Design review of the part built by this model. Coordinates are the model's own, in mm. A direction names the side the tool comes from. Round coordinates to 2 decimals unless told otherwise and drop trailing zeros. Loops run counter-clockwise (first coordinate to the right, second up) from the corner with the lowest first, then second, coordinate; pieces in that order, holes last. Notation, with made-up numbers: (-3.5, 12.5) - (7.5, 12.5) arc R18 ccw to (7.5, 30.5) - close; hole circle Ø7 at (11, -31.75). An arc over 180 degrees is marked (long way). Return JSON: item names as keys, results as strings. Group by question number.
from build123d import *

# Parameters (mm, degrees)
SKETCH1_W           = 20
SKETCH1_H           = 82
SKETCH1_R           = 1.25
BOSS_EXTRUDE1_DEPTH = 10
SKETCH2_W           = 20
SKETCH2_H           = 88.9
BOSS_EXTRUDE2_DEPTH = 32
FILLET1_R           = 10
SKETCH3_R           = 2
SKETCH3_R_2         = 3.5
CUT_EXTRUDE1_DEPTH  = 32


with BuildPart() as part:
    # Sketch1 → Boss-Extrude1 (new body)
    with BuildSketch(Plane(origin=(0, 0, 0), x_dir=(1, 0, 0), z_dir=(0, 1, 0))):
        with Locations((10, 35)):
            Rectangle(SKETCH1_W, SKETCH1_H)
        with Locations(Location((5, 46.75, 0), (0, 0, 270))):
            Circle(SKETCH1_R, mode=Mode.SUBTRACT)
        with Locations(Location((15, 46.75, 0), (0, 0, 270))):
            Circle(SKETCH1_R, mode=Mode.SUBTRACT)
        with Locations(Location((5, -2.75, 0), (0, 0, 270))):
            Circle(SKETCH1_R, mode=Mode.SUBTRACT)
        with Locations(Location((15, -2.75, 0), (0, 0, 270))):
            Circle(SKETCH1_R, mode=Mode.SUBTRACT)
    extrude(amount=BOSS_EXTRUDE1_DEPTH)

    # Sketch2 → Boss-Extrude2 (add)
    with BuildSketch(Plane(origin=(0, 0, -76), x_dir=(-1, 0, 0), z_dir=(0, 0, -1))):
        with Locations((-10, 44.45)):
            Rectangle(SKETCH2_W, SKETCH2_H)
    extrude(amount=BOSS_EXTRUDE2_DEPTH)

    # Fillet1
    fillet1_edges = [part.edges().sort_by_distance(p)[0] for p in [
        (10, 10, -76),
    ]]
    fillet(fillet1_edges, radius=FILLET1_R)

    # Sketch3 → Cut-Extrude1 (cut)
    with BuildSketch(Plane(origin=(20, 0, 0), x_dir=(0, 0, -1), z_dir=(1, 0, 0))):
        with Locations((92, 33.136291501)):
            Circle(SKETCH3_R)
        with Locations((103.313708499, 44.45)):
            Circle(SKETCH3_R)
        with Locations((80.686291501, 44.45)):
            Circle(SKETCH3_R)
        with Locations((92, 55.763708499)):
            Circle(SKETCH3_R)
        with Locations((92, 44.45)):
            Circle(SKETCH3_R_2)
    extrude(amount=-CUT_EXTRUDE1_DEPTH, mode=Mode.SUBTRACT)


solid = part.part
Q1. For line 1 (X direction, y = 6.25, z = 2.75); line 2 (Y direction, x = 8.25, z = -92); line 3 (Y direction, x = 7, z = -66.5), list the stretches that pass through material, from the lowest coordinate up.
Q2. Add section B-B, the plane y = 44.45. State the section outline as (x, z) points.
Q3. Add section D-D, the plane z = -92. State the section outline as (x, y) points, plus the area to 3 significant figures.
Q4. Draft analysis for pull direction Y (two halves, no side actions). For faces 1 (the flat face through (10, 10, -31)), 2 (the flat face through (20, 38, -80)), 3 (the cylindrical face through (10.14, 44.538, -101.316)), state which applies: pulls with the +Y half, pulls with the -Y half, needs draft (parallel to the pull), parting line crosses it, or undercut.
Q5. Insertion check: pin 1 Ø1.5 at (x, z) = (16.5, -61.5) entering from +Y; pin 2 Ø3 at (x, z) = (16, -56) entering from -Y; pin 3 Ø1 at (x, y) = (5, 33) entering from +Z. Each pin has a flat end and moves straight along its axis. Give the tip position at first contact, or say it passes through.
Q6. Add section C-C, the plane x = 15. State the section outline as (y, z) points.
Q7. Add section A-A, the plane z = -46.75. State the section outline as (x, y) points.
Q8. Tool access review of faces 4 (the flat face through (10, 55, -76)), 5 (the cylindrical face through (10.14, 33.737, -93.908)): name each direction out of +Z, -Z, +X, -X, +Y, -Y from which nothing blocks a thin tool from reaching the whole face with its end or side.
Evaluation:
{
 "1": {"line 1": "0 to 3.75, 6.25 to 13.75, 16.25 to 20", "line 2": "0 to 31.14, 35.14 to 40.95, 47.95 to 53.76, 57.76 to 88.9", "line 3": "0 to 10.01"},
 "2": {"outline": "(0, -108) - (20, -108) - (20, -105.31) - (0, -105.31) - close; (0, -101.31) - (20, -101.31) - (20, -95.5) - (0, -95.5) - close; (0, -88.5) - (20, -88.5) - (20, -82.69) - (0, -82.69) - close; (0, -78.69) - (20, -78.69) - (20, -76) - (0, -76) - close"},
 "3": {"outline": "(0, 0) - (20, 0) - (20, 31.14) - (0, 31.14) - close; (0, 35.14) - (20, 35.14) - (20, 40.95) - (0, 40.95) - close; (0, 47.95) - (20, 47.95) - (20, 53.76) - (0, 53.76) - close; (0, 57.76) - (20, 57.76) - (20, 88.9) - (0, 88.9) - close", "area": "1,480 mm²"},
 "4": {"face 1": "pulls with the +Y half", "face 2": "needs draft", "face 3": "undercut"},
 "5": {"pin 1": "y = 10", "pin 2": "y = 0", "pin 3": "z = -76"},
 "6": {"outline": "(0, -108) - (88.9, -108) - (88.9, -76) - (20, -76) arc R10 cw to (10, -66) - (10, -48) - (0, -48) - close; (0, -45.5) - (10, -45.5) - (10, 1.5) - (0, 1.5) - close; (0, 4) - (10, 4) - (10, 6) - (0, 6) - close; hole circle Ø4 at (33.14, -92); hole circle Ø7 at (44.45, -92); hole circle Ø4 at (44.45, -103.31); hole circle Ø4 at (44.45, -80.69); hole circle Ø4 at (55.76, -92)"},
 "7": {"outline": "(0, 0) - (3.75, 0) - (3.75, 10) - (0, 10) - close; (6.25, 0) - (13.75, 0) - (13.75, 10) - (6.25, 10) - close; (16.25, 0) - (20, 0) - (20, 10) - (16.25, 10) - close"},
 "8": {"face 4": "+Z, +X, -X, +Y", "face 5": "+X, -X"}
}
